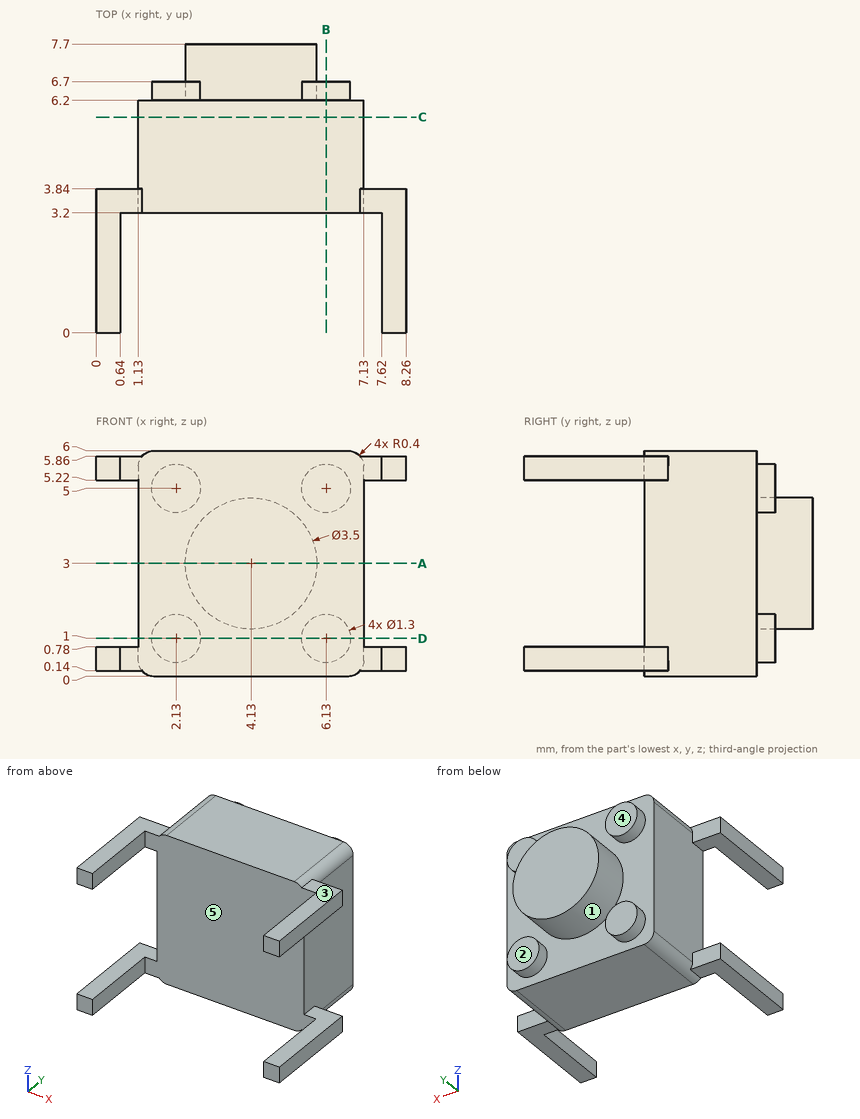
Can you work these out from the drawing? Everything is in mm from the part's minimum corner. A direction names the side the tool comes from. Round coordinates to 2 decimals unless told otherwise and drop trailing zeros. Write each loop counter-clockwise with the first axis right and the second up, starting at its lowest first coordinate (ties: lowest second). Pieces come first, ordered by that corner, then holes.
1. Suppose I cut it at C-C (y = 5.75). List the corners of the cut face in (x, z) for me.
2. Suppose I cut it at A-A (z = 3). List the corners of the cut face in (x, y) for me, and give its area (4 significant figures).
3. If we mould it in two halves opening along X, with no side actions, what happens to the marked faces 1 and 2? For each: released by +X, released by -X, zero draft, split by the parting line, or undercut.
4. I need wall thicknesses on L1, parallel to Z at x = 7.75, y = 2.75; L2, parallel to X at y = 2, z = 0.4; L3, parallel to Y at x = 4.75, z = 2.8. Which ranges of each line are inside material? Lowest first, please.
5. Suppose I cut it at B-B (x = 6.13). List the corners of the cut face in (y, z) for me.
6. For the marked faces 3, 4 and 5, which set-ups out of +Z, -Z, +X, -X, +Y, -Y let a thin tool reach every point of the face, with its end or its side?
7. Will these pins go through, and if not, where does the flat tip stop? pin 1 Ø1.5 at (y, z) = (4.5, 3.5) entering from -X; pin 2 Ø0.9 at (x, y) = (8, 2) entering from +Z; pin 3 Ø0.9 at (x, y) = (1, 2.5) entering from -Z.
8. Suppose I cut it at D-D (z = 1). List the corners of the cut face in (x, y) for me, and give its area (3 significant figures).
Answer sheet:
1. outline: (1.13, 0.4) arc R0.4 ccw to (1.53, 0) - (6.73, 0) arc R0.4 ccw to (7.13, 0.4) - (7.13, 5.6) arc R0.4 ccw to (6.73, 6) - (1.53, 6) arc R0.4 ccw to (1.13, 5.6) - close
2. outline: (1.13, 3.2) - (7.13, 3.2) - (7.13, 6.2) - (5.88, 6.2) - (5.88, 7.7) - (2.38, 7.7) - (2.38, 6.2) - (1.13, 6.2) - close
2. area: 23.25 mm2
3. face 1: undercut
3. face 2: zero draft
4. L1: z = 0.14 to 0.78, 5.22 to 5.86
4. L2: x = 0 to 0.64, 7.62 to 8.26
4. L3: y = 3.2 to 7.7
5. outline: (3.2, 0) - (6.2, 0) - (6.2, 0.35) - (6.7, 0.35) - (6.7, 1.65) - (6.2, 1.65) - (6.2, 4.35) - (6.7, 4.35) - (6.7, 5.65) - (6.2, 5.65) - (6.2, 6) - (3.2, 6) - close
6. face 3: +Z, +X, +Y, -Y
6. face 4: +Z, -X, +Y
6. face 5: +Z, -Z, -Y
7. pin 1: stops at x = 1.13
7. pin 2: stops at z = 5.86
7. pin 3: stops at z = 0.14
8. outline: (1.13, 3.2) - (7.13, 3.2) - (7.13, 6.2) - (6.78, 6.2) - (6.78, 6.7) - (5.48, 6.7) - (5.48, 6.2) - (2.78, 6.2) - (2.78, 6.7) - (1.48, 6.7) - (1.48, 6.2) - (1.13, 6.2) - close
8. area: 19.3 mm2
